```python
from build123d import *

# Parameters (mm, degrees)
ESQUISSE1_W             = 340
ESQUISSE1_H             = 250
BOSS_EXTRU_1_DEPTH      = 6
ESQUISSE10_R            = 2
ESQUISSE10_W            = 6
ESQUISSE10_H            = 7
ESQUISSE10_W_2          = 5
ESQUISSE10_H_2          = 20
ESQUISSE10_W_3          = 21
ESQUISSE10_H_3          = 66
ENL_V_MAT_EXTRU_5_DEPTH = 6
ESQUISSE13_R            = 1.5
ENL_V_MAT_EXTRU_6_DEPTH = 6


with BuildPart() as part:
    # Esquisse1 → Boss.-Extru.1 (new body)
    with BuildSketch(Plane.XY):
        with Locations((-170, 125)):
            Rectangle(ESQUISSE1_W, ESQUISSE1_H)
    extrude(amount=-BOSS_EXTRU_1_DEPTH)

    # Esquisse10 → Enlèv. mat.-Extru.5 (cut)
    with BuildSketch(Plane(origin=(0, 0, -6), x_dir=(-1, 0, 0), z_dir=(0, 0, -1))):
        with Locations((259.9, 45)):
            Circle(ESQUISSE10_R)
        with Locations((259.9, 89)):
            Circle(ESQUISSE10_R)
        with Locations((242.9, 45)):
            Circle(ESQUISSE10_R)
        with Locations((242.9, 89)):
            Circle(ESQUISSE10_R)
        with Locations((215.9, 45)):
            Circle(ESQUISSE10_R)
        with Locations((215.9, 89)):
            Circle(ESQUISSE10_R)
        with Locations(Location((97.1, 89, 0), (0, 0, 180))):
            Circle(ESQUISSE10_R)
        with Locations(Location((97.1, 45, 0), (0, 0, 180))):
            Circle(ESQUISSE10_R)
        with Locations(Location((80.1, 89, 0), (0, 0, 180))):
            Circle(ESQUISSE10_R)
        with Locations(Location((120.1, 89, 0), (0, 0, 180))):
            Circle(ESQUISSE10_R)
        with Locations(Location((120.1, 45, 0), (0, 0, 180))):
            Circle(ESQUISSE10_R)
        with Locations(Location((80.1, 45, 0), (0, 0, 180))):
            Circle(ESQUISSE10_R)
        with Locations((259.9, 35.5)):
            Rectangle(ESQUISSE10_W, ESQUISSE10_H)
        with Locations((259.9, 54.5)):
            Rectangle(ESQUISSE10_W, ESQUISSE10_H)
        with Locations((259.9, 79.5)):
            Rectangle(ESQUISSE10_W, ESQUISSE10_H)
        with Locations((259.9, 98.5)):
            Rectangle(ESQUISSE10_W, ESQUISSE10_H)
        with Locations((242.9, 35.5)):
            Rectangle(ESQUISSE10_W, ESQUISSE10_H)
        with Locations((170, 67)):
            Rectangle(ESQUISSE10_W_2, ESQUISSE10_H_2)
        with Locations((242.9, 54.5)):
            Rectangle(ESQUISSE10_W, ESQUISSE10_H)
        with Locations((242.9, 79.5)):
            Rectangle(ESQUISSE10_W, ESQUISSE10_H)
        with Locations((242.9, 98.5)):
            Rectangle(ESQUISSE10_W, ESQUISSE10_H)
        with Locations((215.9, 35.5)):
            Rectangle(ESQUISSE10_W, ESQUISSE10_H)
        with Locations((215.9, 54.5)):
            Rectangle(ESQUISSE10_W, ESQUISSE10_H)
        with Locations((215.9, 79.5)):
            Rectangle(ESQUISSE10_W, ESQUISSE10_H)
        with Locations((215.9, 98.5)):
            Rectangle(ESQUISSE10_W, ESQUISSE10_H)
        with Locations((97.1, 98.5)):
            Rectangle(ESQUISSE10_W, ESQUISSE10_H)
        with Locations((97.1, 79.5)):
            Rectangle(ESQUISSE10_W, ESQUISSE10_H)
        with Locations((97.1, 54.5)):
            Rectangle(ESQUISSE10_W, ESQUISSE10_H)
        with Locations((97.1, 35.5)):
            Rectangle(ESQUISSE10_W, ESQUISSE10_H)
        with Locations((80.1, 98.5)):
            Rectangle(ESQUISSE10_W, ESQUISSE10_H)
        with Locations((80.1, 79.5)):
            Rectangle(ESQUISSE10_W, ESQUISSE10_H)
        with Locations((120.1, 98.5)):
            Rectangle(ESQUISSE10_W, ESQUISSE10_H)
        with Locations((120.1, 79.5)):
            Rectangle(ESQUISSE10_W, ESQUISSE10_H)
        with Locations((80.1, 54.5)):
            Rectangle(ESQUISSE10_W, ESQUISSE10_H)
        with Locations((120.1, 54.5)):
            Rectangle(ESQUISSE10_W, ESQUISSE10_H)
        with Locations((120.1, 35.5)):
            Rectangle(ESQUISSE10_W, ESQUISSE10_H)
        with Locations((80.1, 35.5)):
            Rectangle(ESQUISSE10_W, ESQUISSE10_H)
        with Locations((282.4, 67)):
            Rectangle(ESQUISSE10_W_3, ESQUISSE10_H_3)
        with Locations((57.6, 67)):
            Rectangle(ESQUISSE10_W_3, ESQUISSE10_H_3)
    extrude(amount=-ENL_V_MAT_EXTRU_5_DEPTH, mode=Mode.SUBTRACT)

    # Esquisse13 → Enlèv. mat.-Extru.6 (cut)
    with BuildSketch(Plane(origin=(0, 0, -6), x_dir=(-1, 0, 0), z_dir=(0, 0, -1))):
        with Locations((69.249793531, 190.11516604)):
            Circle(ESQUISSE13_R)
        with Locations((119.624896765, 190.11516604)):
            Circle(ESQUISSE13_R)
        with Locations(Location((220.375103235, 190.11516604, 0), (0, 0, 180))):
            Circle(ESQUISSE13_R)
        with Locations(Location((270.750206469, 190.11516604, 0), (0, 0, 180))):
            Circle(ESQUISSE13_R)
        with Locations((27, 27)):
            Circle(ESQUISSE13_R)
        with Locations((130, 62.4)):
            Circle(ESQUISSE13_R)
        with Locations(Location((210, 62.4, 0), (0, 0, 180))):
            Circle(ESQUISSE13_R)
        with Locations((37, 27)):
            Circle(ESQUISSE13_R)
        with Locations(Location((37, 107.148940914, 0), (0, 0, 180))):
            Circle(ESQUISSE13_R)
        with Locations(Location((27, 107.148940914, 0), (0, 0, 180))):
            Circle(ESQUISSE13_R)
        with Locations(Location((303, 27, 0), (0, 0, 180))):
            Circle(ESQUISSE13_R)
        with Locations(Location((313, 27, 0), (0, 0, 180))):
            Circle(ESQUISSE13_R)
        with Locations((313, 107.148940914)):
            Circle(ESQUISSE13_R)
        with Locations((303, 107.148940914)):
            Circle(ESQUISSE13_R)
        Polygon((43, 100), (21, 100), (21, 90), (14, 90), (14, 44), (21, 44), (21, 34), (43, 34), (43, 38.074470457), (47.1, 38.074470457), (47.1, 96.074470457), (43, 96.074470457), align=None)
        Polygon((297, 38.074470457), (297, 34), (319, 34), (319, 44), (326, 44), (326, 90), (319, 90), (319, 100), (297, 100), (297, 96.074470457), (292.9, 96.074470457), (292.9, 38.074470457), align=None)
    extrude(amount=-ENL_V_MAT_EXTRU_6_DEPTH, mode=Mode.SUBTRACT)


solid = part.part
```
Read the model definition and answer for the solid it produces. Units are mm, in the model's axes. Give positions to 0.01 mm unless a question says otherwise; leave off trailing zeros. One line per item, written item: value. Start each with the question number.
(1) The part is cut by section A-A (z = -1.3). State how many separate pieces and enclosed holes the cut face has, and give its area (3 significant figures).
(2) Straight lines are drawn through the part: L1, parallel to Y at x = -313, z = -2.25; L2, parallel to Y at x = -240, z = -0.5; L3, parallel to Y at x = -274, z = -1.25. For each, find the intervals that lie inside material, in ascending order.
(3) A flat-ended cylindrical pin translates along its axis: P1, Ø3.5, axis at x = -120.1, y = 45, coming from the +Z side. Find the tip coordinate at first contact, or state that the pin passes through.
Taken from the geometry:
1. separate pieces: 1
1. enclosed holes: 53
1. area: 76,800 mm^2
2. L1: 0 to 25.5, 28.5 to 34, 100 to 105.65, 108.65 to 250
2. L2: 0 to 32, 39 to 51, 58 to 76, 83 to 95, 102 to 250
2. L3: 0 to 34, 100 to 250
3. P1: through
